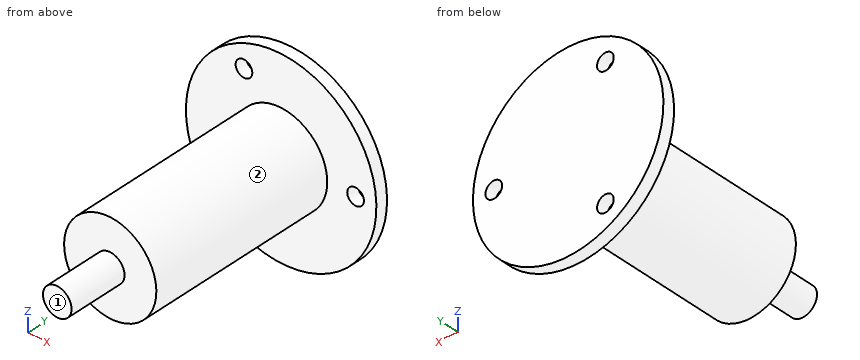
from build123d import *

# Parameters (mm, degrees)
CUT_EXTRUDE1_DEPTH      = 41.924442574
CUT_EXTRUDE1_DEPTH_BACK = 41.924442574
SKETCH2_R               = 1.4
SKETCH4_R               = 2.4


# Read off the part's stored shape, not the designer's step: Split2
with BuildPart() as part:
    # Sketch1 → Revolve1 (revolve)
    with BuildSketch(Plane(origin=(0, 0, 0), x_dir=(0, 0, -1), z_dir=(1, 0, 0)), mode=Mode.PRIVATE) as revolve1_sk:
        Polygon((0, 20.05), (2.95, 20.05), (2.95, 14.05), (16, 14.05), (16, 12.05), (7.75, 12.05), (7.75, -20.05), (0, -20.05), align=None)
    revolve(revolve1_sk.sketch.rotate(Axis((0, 23.931122449, 0), (0, -1, 0)), 180), axis=Axis((0, 23.931122449, 0), (0, -1, 0)))

    # Sketch2 → Cut-Extrude1 (cut, two sides: drawn at the far end of the back side and taken through both)
    with BuildSketch(Plane(origin=(0, 14.05, 0), x_dir=(1, 0, 0), z_dir=(0, 1, 0)).offset(-CUT_EXTRUDE1_DEPTH_BACK)):
        with Locations(Location((12.5, 0, 0), (0, 0, 270))):
            Circle(SKETCH2_R)
        with Locations(Location((-6.25, -10.825317547, 0), (0, 0, 270))):
            Circle(SKETCH2_R)
        with Locations(Location((-6.25, 10.825317547, 0), (0, 0, 270))):
            Circle(SKETCH2_R)
    extrude(amount=CUT_EXTRUDE1_DEPTH + CUT_EXTRUDE1_DEPTH_BACK, mode=Mode.SUBTRACT)

    # Sweep1: sweep along a path in Sketch5
    with BuildLine(Plane(origin=(0, 0, 0), x_dir=(0, 0, -1), z_dir=(1, 0, 0))) as sweep1_path:
        Line((30, 52.05), (30, 32.05))
        ThreePointArc((30, 32.05), (28.242640687, 27.807359313), (24, 26.05))
        Line((24, 26.05), (6, 26.05))
        ThreePointArc((6, 26.05), (1.757359313, 24.292640687), (0, 20.05))
        Line((0, 20.05), (0, 0))
        Line((0, 0), (0, -30))
    # Sketch4 → Sweep1 (sweep)
    with BuildSketch(Plane(origin=(0, 0, 0), x_dir=(1, 0, 0), z_dir=(0, 1, 0))):
        Circle(SKETCH4_R)
    sweep(path=sweep1_path.line)


with BuildPart() as body_2:
    # Split2: the piece on the far side of the plane
    add(part.part)
    split(bisect_by=Plane(origin=(0, 14.05, 0), x_dir=(1, 0, 0), z_dir=(0, 1, 0)), keep=Keep.BOTTOM)


with BuildPart() as part_1:
    add(part.part)

    # Split2
    split(bisect_by=Plane(origin=(0, 14.05, 0), x_dir=(1, 0, 0), z_dir=(0, 1, 0)), keep=Keep.TOP)


solid = body_2.part
Here's how the part is built. I have some questions about the finished solid (model axes, mm). Face numbers are marked on the shaded views. A direction names the side the tool comes from. Give positions to 0.01 mm unless a question says otherwise; leave off trailing zeros. Loops run counter-clockwise (first coordinate to the right, second up) from the corner with the lowest first, then second, coordinate; pieces in that order, holes last. Notation, with made-up numbers: (64, 31.5) -> (92, 31.5) arc R29 ccw to (92, 68.5) -> close; hole circle Ø11 at (-10, -6). An arc over 180 degrees is marked (long way). Answer as a JSON object with one key per item and string values. Group by question number.
Item 1: On a 3-axis mill with a long thin cutter (end or side, diameter ignored), from which of +Z, -Z, +X, -X, +Y, -Y can I reach the whole of each face in a straight line? I mean the marked faces 1 and 2. Say none if no direction works.
Item 2: Imagine slicing it at A-A on z = 0. Write out the boundary of the cut face in (x, y).
Item 3: I need wall thicknesses on L1, parallel to Z at x = -6.25, y = 13; L2, parallel to Z at x = -6, y = 13; L3, parallel to X at y = 13.4, z = 0. Which ranges of each line are inside material? Lowest first, please.
Item 4: Will these pins go through, and if not, where does the flat tip stop? pin 1 (1.5 mm diameter, centred on x = 11, z = 11.5, fed in from -Y); pin 2 (3 mm diameter, centred on x = 0, y = 1, fed in from -Z); pin 3 (1 mm diameter, centred on y = -7.5, z = 9, fed in from -X); pin 4 (5 mm diameter, centred on y = 2, z = -3.5, fed in from +X).
Item 5: Imagine slicing it at C-C on x = 0. Write out the boundary of the cut face in (y, z).
Item 6: Imagine slicing it at B-B on x = 12.5. Write out the boundary of the cut face in (y, z), then the cut area to 4 significant figures.
Item 7: Imagine slicing it at D-D on y = -12. Write out the boundary of the cut face in (x, z).
Answer list:
{
 "1": {"face 1": "+Z, -Z, +X, -X, -Y", "face 2": "-Y"},
 "2": {"outline": "(-16, 12.05) -> (-7.75, 12.05) -> (-7.75, -20.05) -> (-2.4, -20.05) -> (-2.4, -30) -> (2.4, -30) -> (2.4, -20.05) -> (7.75, -20.05) -> (7.75, 12.05) -> (11.1, 12.05) -> (11.1, 14.05) -> (-16, 14.05) -> close; (13.9, 12.05) -> (16, 12.05) -> (16, 14.05) -> (13.9, 14.05) -> close"},
 "3": {"L1": "z = -14.73 to -12.23, -9.43 to 9.43, 12.23 to 14.73", "L2": "z = -14.83 to -12.2, -9.45 to 9.45, 12.2 to 14.83", "L3": "x = -16 to 11.1, 13.9 to 16"},
 "4": {"pin 1": "stops at y = 12.05", "pin 2": "stops at z = -7.75", "pin 3": "passes through", "pin 4": "stops at x = 7.69"},
 "5": {"outline": "(-30, -2.4) -> (-20.05, -2.4) -> (-20.05, -7.75) -> (12.05, -7.75) -> (12.05, -16) -> (14.05, -16) -> (14.05, 16) -> (12.05, 16) -> (12.05, 7.75) -> (-20.05, 7.75) -> (-20.05, 2.4) -> (-30, 2.4) -> close"},
 "6": {"outline": "(12.05, -9.99) -> (14.05, -9.99) -> (14.05, -1.4) -> (12.05, -1.4) -> close; (12.05, 1.4) -> (14.05, 1.4) -> (14.05, 9.99) -> (12.05, 9.99) -> close", "area": "34.35 mm2"},
 "7": {"outline": "circle Ø15.5 at (0, 0)"}
}
